from build123d import *

# Parameters (mm, degrees)
BOSS_EXTRUDE1_DEPTH = 7
BOSS_EXTRUDE2_START = -2
SKETCH2_R           = 1.9
BOSS_EXTRUDE2_DEPTH = 2
BOSS_EXTRUDE3_START = -5
BOSS_EXTRUDE3_DEPTH = 5
SKETCH4_R           = 1.9
CUT_EXTRUDE1_DEPTH  = 5
BOSS_EXTRUDE4_START = -5
BOSS_EXTRUDE4_DEPTH = 5
SKETCH6_R           = 1.9
CUT_EXTRUDE2_DEPTH  = 4


with BuildPart() as part:
    # Sketch1 → Boss-Extrude1 (new body)
    with BuildSketch(Plane.XY):
        with BuildLine():
            Line((-3.636312194, 12.481075019), (-3.21673771, 11.040950978))
            ThreePointArc((-3.21673771, 11.040950978), (1.401778308, -11.414246255), (0.449573558, 11.491208971))
            Line((0.449573558, 11.491208971), (0.449573558, 12.992223967))
            ThreePointArc((0.449573558, 12.992223967), (1.613736067, -12.899451768), (-3.636312194, 12.481075019))
        make_face()
    extrude(amount=-BOSS_EXTRUDE1_DEPTH)

    # Sketch2 → Boss-Extrude2 (add)
    # profile 1 of 6: a face of its own
    with BuildSketch(Plane(origin=(0, 0, -7), x_dir=(-1, 0, 0), z_dir=(0, 0, -1)).offset(BOSS_EXTRUDE2_START)):
        Polygon((13, -1.4e-08), (13, -3), (17.8, -3), (17.8, 3), (13, 3), align=None)
        with Locations((15.4, 0)):
            Circle(SKETCH2_R, mode=Mode.SUBTRACT)
    # profile 2 of 6: a face of its own
    with BuildSketch(Plane(origin=(0, 0, -7), x_dir=(-1, 0, 0), z_dir=(0, 0, -1)).offset(BOSS_EXTRUDE2_START)):
        with BuildLine():
            ThreePointArc((13, -1.4e-08), (12.911979676, -1.510225432), (12.649110641, -3))
            Line((12.649110641, -3), (13, -3))
            Line((13, -3), (13, -1.4e-08))
        make_face()
    # profile 3 of 6: a face of its own
    with BuildSketch(Plane(origin=(0, 0, -7), x_dir=(-1, 0, 0), z_dir=(0, 0, -1)).offset(BOSS_EXTRUDE2_START)):
        with BuildLine():
            ThreePointArc((12.649110641, 3), (12.911979677, 1.510225419), (13, -1.4e-08))
            Line((13, -1.4e-08), (13, 3))
            Line((13, 3), (12.649110641, 3))
        make_face()
    # profile 4 of 6: a face of its own
    with BuildSketch(Plane(origin=(0, 0, -7), x_dir=(-1, 0, 0), z_dir=(0, 0, -1)).offset(BOSS_EXTRUDE2_START)):
        Polygon((-17.8, -3), (-13, -3), (-13, 2e-09), (-13, 3), (-17.8, 3), align=None)
        with Locations((-15.4, 0)):
            Circle(SKETCH2_R, mode=Mode.SUBTRACT)
    # profile 5 of 6: a face of its own
    with BuildSketch(Plane(origin=(0, 0, -7), x_dir=(-1, 0, 0), z_dir=(0, 0, -1)).offset(BOSS_EXTRUDE2_START)):
        with BuildLine():
            Line((-13, -3), (-12.649110641, -3))
            ThreePointArc((-12.649110641, -3), (-12.911979677, -1.510225425), (-13, 2e-09))
            Line((-13, 2e-09), (-13, -3))
        make_face()
    # profile 6 of 6: a face of its own
    with BuildSketch(Plane(origin=(0, 0, -7), x_dir=(-1, 0, 0), z_dir=(0, 0, -1)).offset(BOSS_EXTRUDE2_START)):
        with BuildLine():
            Line((-13, 3), (-13, 2e-09))
            ThreePointArc((-13, 2e-09), (-12.911979676, 1.510225426), (-12.649110641, 3))
            Line((-12.649110641, 3), (-13, 3))
        make_face()
    extrude(amount=BOSS_EXTRUDE2_DEPTH)

    # Sketch3 → Boss-Extrude3 (add)
    with BuildSketch(Plane(origin=(0, 0, -7), x_dir=(-1, 0, 0), z_dir=(0, 0, -1)).offset(BOSS_EXTRUDE3_START)):
        with BuildLine():
            Line((-1.717517475, 17.992223967), (-0.449573558, 17.992223967))
            Line((-0.449573558, 17.992223967), (-0.449573558, 13))
            Line((-0.449573558, 13), (-2.717517475, 13))
            Line((-2.717517475, 13), (-2.717517475, 16.992223967))
            ThreePointArc((-2.717517475, 16.992223967), (-2.424624256, 17.699330748), (-1.717517475, 17.992223967))
        make_face()
        with BuildLine():
            Line((-0.595067825, 12.986373408), (-2.717517475, 12.889117574))
            Line((-2.717517475, 12.889117574), (-2.717517475, 12.712792721))
            ThreePointArc((-2.717517475, 12.712792721), (-1.661931689, 12.893330953), (-0.595067825, 12.986373408))
        make_face()
        Polygon((-2.717517475, 13), (-2.717517475, 12.889117574), (-0.595067825, 12.986373408), (-0.449573558, 12.993040311), (-0.449573558, 13), align=None)
    extrude(amount=BOSS_EXTRUDE3_DEPTH)

    # Sketch4 → Cut-Extrude1 (cut)
    with BuildSketch(Plane(origin=(2.717517475, 0, 0), x_dir=(0, 0, -1), z_dir=(1, 0, 0))):
        with Locations(Location((4.533929619, 14.83079483, 0), (0, 0, 90))):
            Circle(SKETCH4_R)
    extrude(amount=-CUT_EXTRUDE1_DEPTH, mode=Mode.SUBTRACT)

    # Sketch5 → Boss-Extrude4 (add)
    with BuildSketch(Plane(origin=(0, 0, -7), x_dir=(-1, 0, 0), z_dir=(0, 0, -1)).offset(BOSS_EXTRUDE4_START)):
        with BuildLine():
            Line((5.034893807, 17.281488488), (3.691292994, 12.669788048))
            Line((3.691292994, 12.669788048), (4.784802098, 12.133026974))
            Line((4.784802098, 12.133026974), (5.907276717, 15.985746207))
            ThreePointArc((5.907276717, 15.985746207), (5.823864315, 16.746554204), (5.226910346, 17.225545223))
            Line((5.226910346, 17.225545223), (5.034893807, 17.281488488))
        make_face()
        with BuildLine():
            Line((4.784802098, 12.133026974), (3.691292994, 12.669788048))
            Line((3.691292994, 12.669788048), (3.636312194, 12.481075019))
            ThreePointArc((3.636312194, 12.481075019), (4.209094298, 12.299736793), (4.772886303, 12.092127866))
            Line((4.772886303, 12.092127866), (4.784802098, 12.133026974))
        make_face()
    extrude(amount=BOSS_EXTRUDE4_DEPTH)

    # Sketch6 → Cut-Extrude2 (cut)
    with BuildSketch(Plane(origin=(-1.152099233, -0.335659587, 0), x_dir=(0, 0, 1), z_dir=(-0.9600826937679848, -0.2797163225970375, 0))):
        with Locations(Location((-4.412219036, 15.262129774, 0), (0, 0, 66.15869914))):
            Circle(SKETCH6_R)
    extrude(amount=-CUT_EXTRUDE2_DEPTH, mode=Mode.SUBTRACT)


solid = part.part
Read the model definition and answer for the solid it produces. Units are mm, in the model's axes. A direction names the side the tool comes from. Give positions to 0.01 mm unless a question says otherwise; leave off trailing zeros. Loops run counter-clockwise (first coordinate to the right, second up) from the corner with the lowest first, then second, coordinate; pieces in that order, holes last. Notation, with made-up numbers: (52, 31.5) - (89, 31.5) arc R29 cw to (89, 65.5) - close; hole circle Ø3 at (87, 19). An arc over 180 degrees is marked (long way). Answer as CSV lines item,"result". Start each with the question number.
1) Find section A-A (x = -15.4). Write down the section's boundary in (y, z), then the cut area to 3 significant figures.
2) Find section D-D (z = -3.25). Write down the section's boundary in (x, y).
3) Which of the six approach directions +Z, -Z, +X, -X, +Y, -Y give full straight-line access (tool end or side, diameter ignored) to faces 4 (the face through (15, -3, -6)), 5 (the face through (2.718, 16.8, -3.9)), 6 (the face through (-15, 3, -6)), 7 (the face through (0.45, 17, -4))?
4) Find section C-C (y = -5). Write down the section's boundary in (x, z).
5) Straight lines are drawn through the part: L1, parallel to Y at x = 15.4, z = -5.45; L2, parallel to X at y = 1, z = -5.5; L3, parallel to Y at x = -6.5, z = -4.5. For each, find the intervals that lie inside material, in ascending order. Write a range as from..to.
6) Determine the mould class of faces 1 (the face through (1.599, 16.586, -5.262)), 2 (the face through (2.432, 17.692, -4.465)), 3 (the face through (1, 12, -7)) for opening direction Z: released by +Z, released by -Z, zero draft, split by the parting line, or undercut.
7) Find section B-B (y = 0). Write down the section's boundary in (x, z).
8) Each of these flat-tipped pins is pushed along its axis until it touches: pin 1 Ø1.5 at (x, z) = (12.5, -2.5) entering from -Y; pin 2 Ø1 at (x, z) = (15, -5.5) entering from -Y; pin 3 Ø3.5 at (y, z) = (15, -3.5) entering from +X. Where does it stop, or does it pass through?
Findings below:
1,outline,"(-3, -7) - (-1.9, -7) - (-1.9, -5) - (-3, -5) - close; (1.9, -7) - (3, -7) - (3, -5) - (1.9, -5) - close"
1,area,"4.40 mm^2"
2,outline,"(-5.91, 15.99) - (-5.84, 15.76) - (-4.69, 16.1) - (-5.03, 17.28) - (-5.23, 17.23) arc R1 ccw to start; (-5, 12.87) - (-4.77, 12.09) arc R13 ccw (long way) to (2.72, 12.71) - (2.72, 13.43) - (0.45, 13.43) - (0.45, 12.99) - (0.6, 12.99) arc R13 ccw to (0.45, 12.99) - (0.45, 11.49) arc R11.5 cw (long way) to (-3.22, 11.04) - (-3.85, 13.21) - close; (0.45, 16.23) - (2.72, 16.23) - (2.72, 16.99) arc R1 ccw to (1.72, 17.99) - (0.45, 17.99) - close"
3,face 4,"+Z, -Z, +X, -Y"
3,face 5,"+Z, -Z, +X, +Y"
3,face 6,"+Z, -Z, -X, +Y"
3,face 7,"+Z, -Z, +Y"
4,outline,"(-12, -7) - (-10.36, -7) - (-10.36, 0) - (-12, 0) - close; (10.36, -7) - (12, -7) - (12, 0) - (10.36, 0) - close"
5,L1,"-3..-1.9, 1.9..3"
5,L2,"-17.8..-17.02, -13.78..-11.46, 11.46..13.78, 17.02..17.8"
5,L3,"-11.26..-9.49, 9.49..11.26"
6,face 1,"undercut"
6,face 2,"zero draft"
6,face 3,"released by -Z"
7,outline,"(-17.8, -7) - (-17.3, -7) - (-17.3, -5) - (-17.8, -5) - close; (-13.5, -7) - (-11.5, -7) - (-11.5, 0) - (-13, 0) - (-13, -5) - (-13.5, -5) - close; (11.5, -7) - (13.5, -7) - (13.5, -5) - (13, -5) - (13, 0) - (11.5, 0) - close; (17.3, -7) - (17.8, -7) - (17.8, -5) - (17.3, -5) - close"
8,pin 1,"y = -5.56"
8,pin 2,"y = -3"
8,pin 3,"x = 2.72"
